Model file for the job. Use its own axes, mm. A direction names the side the tool comes from. Coordinates: 2 decimals unless noted, no trailing zeros. One line per question, with ' | ' between items. Start each with the question number.
(1) Wall check: probe 1 along Y at (x, z) = (0, 0.8); probe 2 along Z at (x, y) = (-2.75, 2.25); probe 3 along X at (y, z) = (-3.5, 3.5). Give the ranges that are in metal, low to high.
(2) Tool access for faces 4 (the face through (-0.27, -1.22, 1.27)), 5 (the face through (2.14, 3.74, 5.21)): list every direction of +Z, -Z, +X, -X, +Y, -Y with a clear straight run to the whole face (end or side of a thin tool).
(3) Two-plate mould, pull along X, no slides. Class faces 1 (the face through (-2, 0, 0)), 2 (the face through (-2.17, -9.76, 1.3)), 3 (the face through (-3.47, -1.99, 5.29)): +X half, -X half, draft (parallel to the pull), parting line (faces both ways), or undercut.
(4) Flat gauge pins, fed straight in: pin 1 Ø4 at (x, y) = (1.5, 1) entering from +Z; pin 2 Ø1.8 at (x, z) = (-0.5, 5) entering from -Y; pin 3 Ø2 at (x, z) = (7, 5.5) entering from +Y. Where does each tip first touch, or does it go through?
from build123d import *

# Parameters (mm, degrees)
F3_DEPTH = 5.5
F4_R     = 1.25
F5_DEPTH = 3
F6_R     = 2


with BuildPart() as f1:
    # F0 (on Front) → F1 (revolve)
    with BuildSketch(Plane.XZ):
        with BuildLine():
            Line((0, 8), (0, 0))
            Line((0, 0), (10, 0))
            Line((10, 0), (10, 2.567338))
            ThreePointArc((10, 2.567338), (9.705546, 4.25785), (8.856867, 5.749252))
            Line((8.856867, 5.749252), (7, 8))
            Line((7, 8), (0, 8))
        make_face()
    revolve(axis=Axis((0, 0, 6.785496), (0, 0, 1)))

    # F2 (on face) → F3 (cut)
    with BuildSketch(Plane.XY.offset(8)):
        Polygon((2.309401, 4), (-2.309401, 4), (-4.618802, 0), (-2.309401, -4), (2.309401, -4), (4.618802, 0), align=None)
    extrude(amount=-F3_DEPTH, mode=Mode.SUBTRACT)

    # F4 (on face) → F5 (cut)
    with BuildSketch(Plane.XY.offset(2.5)):
        Circle(F4_R)
    extrude(amount=-F5_DEPTH, mode=Mode.SUBTRACT)

    # F6
    f6_edges = [f1.edges().sort_by_distance(p)[0] for p in [
        (-2.309401, 4, 5.25),
        (2.309401, 4, 5.25),
        (-2.309401, -4, 5.25),
        (2.309401, -4, 5.25),
        (-4.618802, 0, 5.25),
        (4.618802, 0, 5.25),
    ]]
    fillet(f6_edges, radius=F6_R)


solid = f1.part
Filled in:
1) probe 1: -10 to -1.25, 1.25 to 10 | probe 2: 0 to 2.5 | probe 3: -9.27 to -2.48, 2.48 to 9.27
2) face 4: +Z, -Z | face 5: +Z
3) face 1: draft | face 2: parting line | face 3: undercut
4) pin 1: z = 2.5 | pin 2: y = -9.75 | pin 3: y = 7.1
